Here's how the part is built. I have some questions about the finished solid (model axes, mm). Face numbers are marked on the shaded views. A direction names the side the tool comes from. Give positions to 0.01 mm unless a question says otherwise; leave off trailing zeros. Write each loop counter-clockwise with the first axis right and the second up, starting at its lowest first coordinate (ties: lowest second). Pieces come first, ordered by that corner, then holes. Notation, with made-up numbers: (79.25, 47) - (133.25, 47) arc R30 cw to (133.25, 85) - close; hole circle Ø9 at (45, 20.25). An arc over 180 degrees is marked (long way). One line per item, written item: value. Start each with the question number.
1) We'd pull the mould along X, two halves only. Please class the marked faces 4, 5 and 6: +X half, -X half, draft (parallel to the pull), parting line (faces both ways), or undercut.
2) Imagine slicing it at A-A on z = 66. Write out the boundary of the cut face in (x, y), plus the area to 3 significant figures.
3) I'm going to push flat-ended pins straight in: P1, Ø3, axis at y = -2, z = 17.5, coming from the -X side; P2, Ø12, axis at x = 12.5, z = 82.5, coming from the +Y side; P3, Ø10, axis at x = 100, z = 44, coming from the -Y side; P4, Ø4, axis at x = -0.5, z = 81.5, coming from the -Y side. Where does each tip first touch, or does it pass through?
4) Imagine slicing it at C-C on z = 81. Write out the boundary of the cut face in (x, y).
5) Imagine slicing it at B-B on x = 105. Write out the boundary of the cut face in (y, z), plus the area to 3 significant figures.
6) On a 3-axis mill with a long thin cutter (end or side, diameter ignored), from which of +Z, -Z, +X, -X, +Y, -Y can I reach the whole of each face in a straight line? I mean the marked faces 1, 2 and 3. Say none if no direction works.
7) Please list where these lines run through material, in increasing order: L1, parallel to Z at x = 21, y = 12.5; L2, parallel to Y at x = 9, z = 14.5; L3, parallel to X at y = -22.5, z = 44.5. Write a range as [from, to].
from build123d import *

# Parameters (mm, degrees)
F1_DEPTH = 74.9415531754
F2_R     = 5.08
F3_R     = 6.5155077524
F4_DEPTH = 24.241162464
F6_DEPTH = 25
F7_R     = 5
F8_DEPTH = 25
F9_DEPTH = 40.1649922132


with BuildPart() as f1:
    # F0 (on Top) → F1 (new body)
    with BuildSketch(Plane.XY):
        Polygon((38.1590723991, -25.1938253641), (26.3724923134, 35.654425621), (-32.413110137, -50.5349785089), align=None)
    extrude(amount=F1_DEPTH)

    # F2
    f2_edges = [f1.edges().sort_by_distance(p)[0] for p in [
        (2.872981, -37.864402, 74.941553),
        (32.265782, 5.2303, 74.941553),
        (38.159072, -25.193825, 37.470777),
    ]]
    fillet(f2_edges, radius=F2_R)

    # F3 (on face) → F4 (join)
    with BuildSketch(Plane.XY.offset(74.9415531754)):
        with Locations((8.9773815125, -11.1496802419)):
            Circle(F3_R)
    extrude(amount=F4_DEPTH)

    # F5 (on face) → F6 (join)
    with BuildSketch(Plane(origin=(32.0754000375, 6.2131493544, 0), x_dir=(-0.1901696352, 0.9817512464, 0), z_dir=(0.9817512464, 0.1901696352, 0))):
        Polygon((0, 57.1491196752), (-19.9005380273, 27.401227504), (12.399494648, 24.3145730346), align=None)
    extrude(amount=F6_DEPTH)

    # F7
    f7_edges = [f1.edges().sort_by_distance(p)[0] for p in [
        (55.440178, 17.054, 40.731846),
        (57.332417, 7.285311, 25.8579),
        (58.51142, 1.198701, 42.275174),
    ]]
    fillet(f7_edges, radius=F7_R)

    # F8 (add): a face of the model
    f8_faces = [f1.faces().sort_by_distance(p)[0] for p in [
        (57.091234066, 8.5304160504, 35.9772892723),
    ]]
    extrude(f8_faces, amount=F8_DEPTH)

    # F9 (add): a face of the model
    f9_faces = [f1.faces().sort_by_distance(p)[0] for p in [
        (81.6350152267, 13.2846569295, 35.9772892723),
    ]]
    extrude(f9_faces, amount=F9_DEPTH)


solid = f1.part
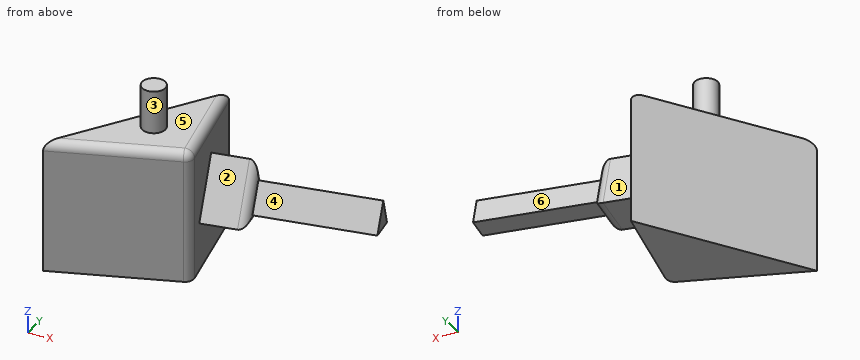
Numbers:
1. face 4: +X half
1. face 5: draft
1. face 6: undercut
2. outline: (-32.41, -50.53) - (34.06, -26.67) arc R5.08 ccw to (37.33, -20.92) - (26.37, 35.65) - close
2. area: 2,290 mm^2
3. P1: x = -0.33
3. P2: y = -4.63
3. P3: y = 13
3. P4: through
4. outline: circle Ø13.03 at (8.98, -11.15)
5. outline: (9.04, 31.58) - (25.32, 30.06) - (19.07, 46.29) - close
5. area: 127 mm^2
6. face 1: +Z, +Y
6. face 2: +Z, +X
6. face 3: +Z
7. L1: [0, 74.94]
7. L2: [-35.66, 10.18]
7. L3: [-13.29, 37.39]
